```python
from build123d import *

# Parameters (mm, degrees)
BOSS_EXTRUDE1_DEPTH  = 8
BOSS_EXTRUDE2_DEPTH  = 2
BOSS_EXTRUDE3_DEPTH  = 5
BOSS_EXTRUDE4_DEPTH  = 3
CUT_EXTRUDE1_DEPTH   = 4
CUT_EXTRUDE2_DEPTH   = 4
BOSS_EXTRUDE5_DEPTH  = 2
BOSS_EXTRUDE6_DEPTH  = 1
BOSS_EXTRUDE7_DEPTH  = 2
BOSS_EXTRUDE8_DEPTH  = 2
CUT_EXTRUDE3_DEPTH   = 1
CUT_EXTRUDE4_DEPTH   = 1
CUT_EXTRUDE5_DEPTH   = 1
CUT_EXTRUDE6_DEPTH   = 1
SKETCH15_W           = 8
SKETCH15_H           = 3.1
CUT_EXTRUDE7_DEPTH   = 4
SKETCH16_W           = 12
SKETCH16_H           = 3
CUT_EXTRUDE8_DEPTH   = 3
SKETCH17_W           = 12
SKETCH17_H           = 3
CUT_EXTRUDE9_DEPTH   = 3
SKETCH18_W           = 6.2
SKETCH18_H           = 6
CUT_EXTRUDE10_DEPTH  = 10.757359313
SKETCH19_W           = 6.2
SKETCH19_H           = 6
CUT_EXTRUDE11_DEPTH  = 10.757359313
BOSS_EXTRUDE9_DEPTH  = 3
SKETCH21_W           = 6.2
SKETCH21_H           = 11
CUT_EXTRUDE12_DEPTH  = 78.756028705
SKETCH22_W           = 6.2
SKETCH22_H           = 11
CUT_EXTRUDE13_DEPTH  = 82.816868676
SKETCH23_W           = 8
SKETCH23_H           = 1
BOSS_EXTRUDE10_DEPTH = 2.8
SKETCH24_W           = 8
SKETCH24_H           = 1
BOSS_EXTRUDE11_DEPTH = 2.8
DRAFT1_START         = -3.1
DRAFT1_DEPTH         = 6.2
DRAFT1_START_2       = -4
DRAFT1_2_DEPTH       = 8
DRAFT2_START         = -3.1
DRAFT2_DEPTH         = 6.2
DRAFT2_START_2       = -4
DRAFT2_2_DEPTH       = 8
RIB1_REACH           = 83.817
SKETCH25_WALL_W      = 177.633737352
SKETCH25_WALL_H      = 1
CHAMFER1_SIZE        = 1
FILLET1_R            = 1


# Read off the part's stored shape, not the designer's step: Draft1, Draft2
with BuildPart() as part:
    # Sketch1 → Boss-Extrude1 (new body)
    with BuildSketch(Plane(origin=(4, 0, 0), x_dir=(0, 0, -1), z_dir=(1, 0, 0))):
        Polygon((-51.757359313, 0), (-10.242640687, 0), (-10.242640687, -9.959797975), (9.959797975, 10.242640687), (0, 10.242640687), (0, 51.757359313), (2.121320344, 53.878679656), (-1, 57), (-5, 57), (-6, 56), (-6, 6), (-56, 6), (-57, 5), (-57, 1), (-53.878679656, -2.121320344), align=None)
    extrude(amount=-BOSS_EXTRUDE1_DEPTH)

    # Sketch2 → Boss-Extrude2 (add)
    with BuildSketch(Plane(origin=(4, 0, 0), x_dir=(0, 0, -1), z_dir=(1, 0, 0))):
        Polygon((0, 4.666904756), (-4.666904756, 0), (-51.757359313, 0), (-53.878679656, -2.121320344), (-57, 1), (-57, 5), (-56, 6), (-6, 6), (-6, 56), (-5, 57), (-1, 57), (2.121320344, 53.878679656), (0, 51.757359313), align=None)
    extrude(amount=BOSS_EXTRUDE2_DEPTH)

    # Sketch3 → Boss-Extrude3 (add)
    with BuildSketch(Plane(origin=(6, 0, 0), x_dir=(0, 0, -1), z_dir=(1, 0, 0))):
        Polygon((-51.757359313, 0), (-53.878679656, -2.121320344), (-57, 1), (-57, 5), (-56, 6), (-6, 6), (-6, 56), (-5, 57), (-1, 57), (2.121320344, 53.878679656), (0, 51.757359313), (0, 0), align=None)
    extrude(amount=BOSS_EXTRUDE3_DEPTH)

    # Sketch4 → Boss-Extrude4 (add)
    with BuildSketch(Plane(origin=(11, 0, 0), x_dir=(0, 0, -1), z_dir=(1, 0, 0))):
        Polygon((-5, 57), (0, 57), (0, 0), (-57, 0), (-57, 5), (-56, 6), (-6, 6), (-6, 56), align=None)
    extrude(amount=BOSS_EXTRUDE4_DEPTH)

    # Sketch5 → Cut-Extrude1 (cut)
    with BuildSketch(Plane(origin=(11, 0, 0), x_dir=(0, 0, -1), z_dir=(1, 0, 0))):
        Polygon((-1, 57), (-3.77594834, 57), (0, 52.5), (0, 51.757359313), (2.121320344, 53.878679656), align=None)
    extrude(amount=-CUT_EXTRUDE1_DEPTH, mode=Mode.SUBTRACT)

    # Sketch6 → Cut-Extrude2 (cut)
    with BuildSketch(Plane(origin=(11, 0, 0), x_dir=(0, 0, -1), z_dir=(1, 0, 0))):
        Polygon((-57, 3.77594834), (-57, 1), (-53.878679656, -2.121320344), (-51.757359313, 0), (-52.5, 0), align=None)
    extrude(amount=-CUT_EXTRUDE2_DEPTH, mode=Mode.SUBTRACT)

    # Sketch7 → Boss-Extrude5 (add)
    with BuildSketch(Plane.ZY.offset(4)):
        Polygon((51.757359313, 0), (4.666904756, 0), (0, 4.666904756), (0, 51.757359313), (-2.121320344, 53.878679656), (1, 57), (5, 57), (6, 56), (6, 6), (56, 6), (57, 5), (57, 1), (53.878679656, -2.121320344), align=None)
    extrude(amount=BOSS_EXTRUDE5_DEPTH)

    # Sketch8 → Boss-Extrude6 (add)
    with BuildSketch(Plane.ZY.offset(6)):
        Polygon((0, 51.757359313), (-2.121320344, 53.878679656), (1, 57), (5, 57), (6, 56), (6, 6), (56, 6), (57, 5), (57, 1), (53.878679656, -2.121320344), (51.757359313, 0), (0, 0), align=None)
    extrude(amount=BOSS_EXTRUDE6_DEPTH)

    # Sketch9 → Boss-Extrude7 (add)
    with BuildSketch(Plane.ZY.offset(7)):
        Polygon((5, 57), (6, 56), (6, 6), (56, 6), (57, 5), (57, 3.77594834), (52.5, 0), (0, 0), (0, 52.5), (3.77594834, 57), align=None)
    extrude(amount=BOSS_EXTRUDE7_DEPTH)

    # Sketch10 → Boss-Extrude8 (add)
    with BuildSketch(Plane.ZY.offset(9)):
        Polygon((0, 0), (0, 52.5), (3.77594834, 57), (5, 57), (57, 5), (57, 3.77594834), (52.5, 0), align=None)
    extrude(amount=BOSS_EXTRUDE8_DEPTH)

    # Sketch11 → Cut-Extrude3 (cut)
    with BuildSketch(Plane.ZY.offset(7)):
        Polygon((53.878679656, -2.121320344), (56, 0), (51.757359313, 0), align=None)
    extrude(amount=-CUT_EXTRUDE3_DEPTH, mode=Mode.SUBTRACT)

    # Sketch12 → Cut-Extrude4 (cut)
    with BuildSketch(Plane(origin=(7, 0, 0), x_dir=(0, 0, -1), z_dir=(1, 0, 0))):
        Polygon((-51.757359313, 0), (-56, 0), (-53.878679656, -2.121320344), align=None)
    extrude(amount=-CUT_EXTRUDE4_DEPTH, mode=Mode.SUBTRACT)

    # Sketch13 → Cut-Extrude5 (cut)
    with BuildSketch(Plane(origin=(7, 0, 0), x_dir=(0, 0, -1), z_dir=(1, 0, 0))):
        Polygon((0, 56), (0, 51.757359313), (2.121320344, 53.878679656), align=None)
    extrude(amount=-CUT_EXTRUDE5_DEPTH, mode=Mode.SUBTRACT)

    # Sketch14 → Cut-Extrude6 (cut)
    with BuildSketch(Plane.ZY.offset(7)):
        Polygon((-2.121320344, 53.878679656), (0, 51.757359313), (0, 56), align=None)
    extrude(amount=-CUT_EXTRUDE6_DEPTH, mode=Mode.SUBTRACT)

    # Sketch15 → Cut-Extrude7 (cut)
    with BuildSketch(Plane(origin=(0, 1.414213562, -1.414213562), x_dir=(-1, 0, 0), z_dir=(0, 0.7071067811865474, -0.7071067811865477))):
        with Locations((0, 1.75)):
            Rectangle(SKETCH15_W, SKETCH15_H)
    extrude(amount=-CUT_EXTRUDE7_DEPTH, mode=Mode.SUBTRACT)

    # Sketch16 → Cut-Extrude8 (cut)
    with BuildSketch(Plane(origin=(0, 25.878679656, 25.878679656), x_dir=(-1, 0, 0), z_dir=(0, -0.707106781186546, -0.7071067811865491))):
        with Locations((0, 38.097979746)):
            Rectangle(SKETCH16_W, SKETCH16_H)
    extrude(amount=-CUT_EXTRUDE8_DEPTH, mode=Mode.SUBTRACT)

    # Sketch17 → Cut-Extrude9 (cut)
    with BuildSketch(Plane(origin=(0, 25.878679656, 25.878679656), x_dir=(-1, 0, 0), z_dir=(0, -0.7071067811865469, -0.7071067811865481))):
        with Locations((0, -38.097979746)):
            Rectangle(SKETCH17_W, SKETCH17_H)
    extrude(amount=-CUT_EXTRUDE9_DEPTH, mode=Mode.SUBTRACT)

    # Sketch18 → Cut-Extrude10 (cut)
    with BuildSketch(Plane.XZ.offset(-10.242640687)):
        with Locations((0, 3)):
            Rectangle(SKETCH18_W, SKETCH18_H)
    extrude(amount=-CUT_EXTRUDE10_DEPTH, mode=Mode.SUBTRACT)

    # Sketch19 → Cut-Extrude11 (cut)
    with BuildSketch(Plane(origin=(0, 0, 10.242640687), x_dir=(-1, 0, 0), z_dir=(0, 0, -1))):
        with Locations((0, 3)):
            Rectangle(SKETCH19_W, SKETCH19_H)
    extrude(amount=-CUT_EXTRUDE11_DEPTH, mode=Mode.SUBTRACT)

    # Sketch20 → Boss-Extrude9 (add)
    with BuildSketch(Plane.ZY.offset(11)):
        Polygon((57, 0), (0, 0), (0, 57), (5, 57), (57, 5), align=None)
    extrude(amount=BOSS_EXTRUDE9_DEPTH)

    # Sketch21 → Cut-Extrude12 (cut, through all)
    with BuildSketch(Plane.XY.offset(6)):
        with Locations((0, 45.5)):
            Rectangle(SKETCH21_W, SKETCH21_H)
    extrude(amount=-CUT_EXTRUDE12_DEPTH, mode=Mode.SUBTRACT)

    # Sketch22 → Cut-Extrude13 (cut, through all)
    with BuildSketch(Plane.XZ):
        with Locations((0, 45.5)):
            Rectangle(SKETCH22_W, SKETCH22_H)
    extrude(amount=-CUT_EXTRUDE13_DEPTH, mode=Mode.SUBTRACT)

    # Sketch23 → Boss-Extrude10 (add)
    with BuildSketch(Plane(origin=(0, 28, 28), x_dir=(-1, 0, 0), z_dir=(0, -0.7071067811865448, -0.7071067811865503))):
        with Locations((0, 39.097979746)):
            Rectangle(SKETCH23_W, SKETCH23_H)
    extrude(amount=BOSS_EXTRUDE10_DEPTH)

    # Sketch24 → Boss-Extrude11 (add)
    with BuildSketch(Plane(origin=(0, 28, 28), x_dir=(-1, 0, 0), z_dir=(0, -0.7071067811865471, -0.7071067811865479))):
        with Locations((0, -39.097979746)):
            Rectangle(SKETCH24_W, SKETCH24_H)
    extrude(amount=BOSS_EXTRUDE11_DEPTH)

    # Draft1 outline → Draft1 (cut)
    with BuildSketch(Plane.YZ.offset(DRAFT1_START)):
        Polygon((0, 40), (0, 34), (6, 40), align=None)
        Polygon((6, 10.242640687), (-9.959797975, 10.242640687), (-1.979898987, 2.2627417), align=None)
    extrude(amount=DRAFT1_DEPTH, mode=Mode.SUBTRACT)

    # Draft1 2 outline → Draft1 2 (cut)
    with BuildSketch(Plane.YZ.offset(DRAFT1_START_2)):
        Polygon((-1.979898987, 2.2627417), (0, 4.242640687), (0, 10.242640687), (-9.959797975, 10.242640687), align=None)
    extrude(amount=DRAFT1_2_DEPTH, mode=Mode.SUBTRACT)

    # Draft2 outline → Draft2 (cut)
    with BuildSketch(Plane.YZ.offset(DRAFT2_START)):
        Polygon((40, 6), (34, 0), (40, 0), align=None)
        Polygon((2.2627417, -1.979898987), (10.242640687, -9.959797975), (10.242640687, 6), align=None)
    extrude(amount=DRAFT2_DEPTH, mode=Mode.SUBTRACT)

    # Draft2 2 outline → Draft2 2 (cut)
    with BuildSketch(Plane.YZ.offset(DRAFT2_START_2)):
        Polygon((4.242640687, 0), (2.2627417, -1.979898987), (10.242640687, -9.959797975), (10.242640687, 0), align=None)
    extrude(amount=DRAFT2_2_DEPTH, mode=Mode.SUBTRACT)

    # Sketch25 wall → Rib1 (add, up to next)
    with BuildSketch(Plane(origin=(0, 1.626345597, 1.626345597), x_dir=(-1, 0, 0), z_dir=(0, 0.707106781187, 0.707106781187)), mode=Mode.PRIVATE) as rib1_sk1:
        Rectangle(SKETCH25_WALL_W, SKETCH25_WALL_H)
    rib1_tool1 = extrude(rib1_sk1.sketch, amount=RIB1_REACH, mode=Mode.PRIVATE) - part.part
    add(rib1_tool1.solids().sort_by_distance((0, 1.626345597, 1.626345597))[0])

    # Chamfer1
    chamfer1_edges = [part.edges().sort_by_distance(p)[0] for p in [
        (12.5, 57, 0),
        (-12.5, 57, 0),
        (-12.5, 0, 57),
        (12.5, 0, 57),
    ]]
    chamfer(chamfer1_edges, length=CHAMFER1_SIZE)

    # Fillet1
    fillet1_edges = [part.edges().sort_by_distance(p)[0] for p in [
        (2.5, 6, 6),
        (-10, 0, 0),
        (10, 0, 0),
    ]]
    fillet(fillet1_edges, radius=FILLET1_R)


solid = part.part
```
Source: CAD feature listing. Evaluate the final solid. Frame: model axes, mm. A direction names the side the tool comes from. Give positions to 0.01 mm unless a question says otherwise; leave off trailing zeros. Write each loop counter-clockwise with the first axis right and the second up, starting at its lowest first coordinate (ties: lowest second). Pieces come first, ordered by that corner, then holes.
1. Pull-direction query (Y, two-part tool) for faces 1 (the face through (-0.056, 1.954, 6.197)), 2 (the face through (7, 55, 1)), 3 (the face through (0.056, -0.269, 54.317)); classes: +Y half, -Y half, draft (parallel to the pull), parting line (faces both ways), or undercut.
2. Section query C-C (x = -12). Return the cut outline in (y, z).
3. Access query for faces 4 (the face through (-3.1, 3, 14)), 5 (the face through (-0.084, 1.224, 3.443)), 6 (the face through (-7, 55, 1)), 7 (the face through (-7, 1, 55)), 8 (the face through (6, 54, 1)). Directions: +Z, -Z, +X, -X, +Y, -Y. A direction counts if a zero-diameter tool reaches every point of the face in a straight line with its end or side. Return the directions, or none.
4. Section query B-B (y = 44.5). Return the cut outline in (x, z).
5. First-contact query: pin 1 (1.5 mm diameter, centred on x = -1.5, y = 30, fed in from -Z); pin 2 (6 mm diameter, centred on x = 9, z = 27, fed in from +Y); pin 3 (1.3 mm diameter, centred on y = -1, z = 55, fed in from +X). Flat tips, straight axial feed; report the tip coordinate or a pass-through.
6. Section query D-D (y = 32.5). Return the cut outline in (x, z).
7. Material intervals for line 1 along X through (y, z) = (5.5, 45); line 2 along Y through (x, z) = (1.5, 5.5); line 3 along X through (y, z) = (10, 14), sorted ascending.
8. Section query A-A (z = 12). Return the cut outline in (x, y), then the cut area to 3 significant figures.
Output values:
1. face 1: -Y half
1. face 2: draft
1. face 3: undercut
2. outline: (0, 1) arc R1 ccw to (1, 0) - (56, 0) - (57, 1) - (57, 5) - (5, 57) - (1, 57) - (0, 56) - close
3. face 4: -Y
3. face 5: none
3. face 6: -Z, +Y
3. face 7: +Z, -Y
3. face 8: -Z
4. outline: (-14, 0) - (-3.1, 0) - (-3.1, 6) - (-9, 6) - (-9, 17.5) - (-14, 17.5) - close; (3.1, 0) - (14, 0) - (14, 6) - (3.1, 6) - close
5. pin 1: stops at z = 0
5. pin 2: stops at y = 6
5. pin 3: stops at x = 4
6. outline: (-14, 0) - (14, 0) - (14, 6) - (-9, 6) - (-9, 29.5) - (-14, 29.5) - close
7. line 1: x = -14 to -3.1, 3.1 to 14
7. line 2: y = 1.26 to 9.74, 21 to 39.5, 51 to 56.5
7. line 3: x = -14 to -9
8. outline: (-14, 0) - (-3.1, 0) - (-3.1, 6) - (-9, 6) - (-9, 50) - (-14, 50) - close; (3.1, 0) - (14, 0) - (14, 6) - (3.1, 6) - close
8. area: 351 mm2
